from build123d import *

# Parameters (mm, degrees)
F0_R     = 11
F2_DEPTH = 2
F1_R     = 3.175
F3_DEPTH = 3


# Not quite as in the source:
# - a fillet or chamfer that OpenCascade refuses, or shapes differently, is made with other operations: its cross-section is extruded or revolved along the edge and cut away or added


with BuildPart() as f2:
    # F0 (on Top) → F2 (new body)
    with BuildSketch(Plane.XY):
        Circle(F0_R)
    extrude(amount=F2_DEPTH)

    # F1 (on Top) → F3 (join)
    with BuildSketch(Plane.XY):
        Circle(F1_R)
    extrude(amount=-F3_DEPTH)

    # F4: fillet of radius 5.08 on 1 edges, made by hand

    # F4_s1 → F4_t2 (revolve, cut)
    with BuildSketch(Plane.XZ):
        with BuildLine():
            ThreePointArc((11, 0), (9.2140835586, 1.4726256161), (6.9601980247, 2))
            Line((6.9601980247, 2), (11, 2))
            Line((11, 2), (11, 0))
        make_face()
    revolve(axis=Axis((0, 0, 2), (0, 0, 1)), mode=Mode.SUBTRACT)


solid = f2.part
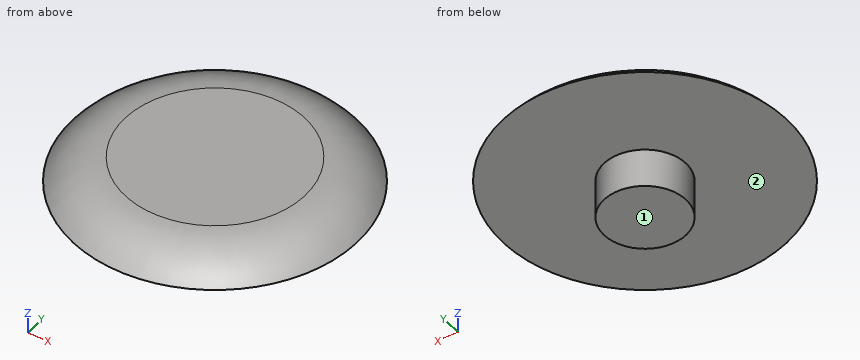
Verification items for the finished model (mm, model axes). Face numbers are marked on the shaded views. A direction names the side the tool comes from. Coordinates: 2 decimals unless noted, no trailing zeros. Write each loop counter-clockwise with the first axis right and the second up, starting at its lowest first coordinate (ties: lowest second). Pieces come first, ordered by that corner, then holes. Notation, with made-up numbers: (55.5, 55.25) - (62.5, 55.25) arc R20 cw to (62.5, 85.25) - close; hole circle Ø8 at (-35.75, -22.75). An arc over 180 degrees is marked (long way). Answer as a JSON object with one key per item and string values.
(1) Cross-section at C-C on z = -1.85. Record the cut outline in (x, y) (3 decimals).
Report:
{"outline": "circle Ø6.35 at (0, 0)"}
(2) Cross-section at D-D on z = 1.15. Record the cut outline in (x, y).
Report:
{"outline": "circle Ø19.55 at (0, 0)"}
(3) Gauge pin test, flat end, axial feed: pin 1 Ø1 at (x, y) = (2, -8.5) entering from +Z. Record the tip position at first contact, or that the pin passes through.
Report:
{"pin 1": "z = 1.84"}
(4) Tool access check on the marked faces 1 and 2. Record the directions out of +Z, -Z, +X, -X, +Y, -Y that give a thin tool (end or side, any length) a straight path to the whole face; none if there is none.
Report:
{"face 1": "-Z, +X, -X, +Y, -Y", "face 2": "-Z"}
(5) Thickness scan on line 1 along Z through (x, y) = (3.75, -1.5); line 2 along Y through (x, z) = (-0.5, -2.1); line 3 along X through (y, z) = (-1, 0.4). Record the ranges inside material, lowest first.
Report:
{"line 1": "0 to 2", "line 2": "-3.14 to 3.14", "line 3": "-10.61 to 10.61"}
(6) Cross-section at A-A on x = 0. Record the cut outline in (y, z) (3 decimals), plus the area to 3 significant figures.
Report:
{"outline": "(-11, 0) - (-3.175, 0) - (-3.175, -3) - (3.175, -3) - (3.175, 0) - (11, 0) arc R5.08 ccw to (6.96, 2) - (-6.96, 2) arc R5.08 ccw to start", "area": "58.2 mm^2"}
